Read the model definition and answer for the solid it produces. Units are mm, in the model's axes. Face numbers are marked on the shaded views. Round coordinates to 2 decimals unless told otherwise and drop trailing zeros. Order: outer loops, then holes, each group sorted by start corner. A loop starts at its lowest first (then second) coordinate and runs counter-clockwise, first axis right, second up.
from build123d import *

# Parameters (mm, degrees)
FILLET_1_R     = 2
FILLET_2_R     = 5
FILLET_3_R     = 7
CHAMFER_1_SIZE = 2
FILLET_4_R     = 1


with BuildPart() as part:
    # Эскиз1 → Повернуть1 (revolve)
    with BuildSketch(Plane.XY, mode=Mode.PRIVATE) as revolve_1_sk:
        Polygon((0, 20), (-11, 20), (-11, 50), (-15, 50), (-17.5, 19), (-22.5, 15), (-22.5, 0), (0, 0), align=None)
    revolve(revolve_1_sk.sketch.rotate(Axis((0, 0, 0), (0, 1, 0)), 270), axis=Axis((0, 0, 0), (0, 1, 0)))

    # Скругление1
    fillet_1_edges = [part.edges().sort_by_distance(p)[0] for p in [
        (0, 50, 15),
    ]]
    fillet(fillet_1_edges, radius=FILLET_1_R)

    # Скругление2
    fillet_2_edges = [part.edges().sort_by_distance(p)[0] for p in [
        (0, 19, 17.5),
    ]]
    fillet(fillet_2_edges, radius=FILLET_2_R)

    # Скругление3
    fillet_3_edges = [part.edges().sort_by_distance(p)[0] for p in [
        (0, 15, 22.5),
    ]]
    fillet(fillet_3_edges, radius=FILLET_3_R)

    # Фаска1
    chamfer_1_edges = [part.edges().sort_by_distance(p)[0] for p in [
        (0, 0, 22.5),
    ]]
    chamfer(chamfer_1_edges, length=CHAMFER_1_SIZE)

    # Скругление4
    fillet_4_edges = [part.edges().sort_by_distance(p)[0] for p in [
        (0, 20, 11),
    ]]
    fillet(fillet_4_edges, radius=FILLET_4_R)


solid = part.part
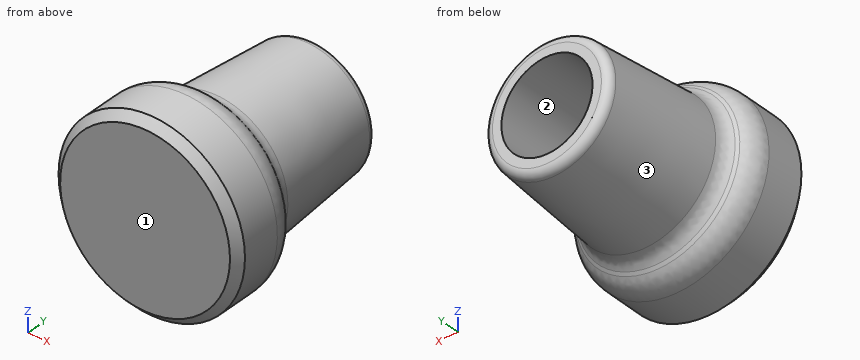
Q1. A cutting plane is placed at A-A, the plane y = 32. Give the vertices of the cut face in (x, z), plus the area to 3 significant figures.
Outcome:
outline: circle Ø32.9 at (0, 0); hole circle Ø22 at (0, 0)
area: 470 mm2
Q2. For a pull along X with two mould halves and no side action, classify the marked faces 1, 2 and 3 as released by +X, released by -X, zero draft, split by the parting line, or undercut.
Outcome:
face 1: zero draft
face 2: undercut
face 3: split by the parting line
Q3. Flat-ended cylindrical pins translate along their axes: pin 1 (5 mm diameter, centred on y = 21.5, z = 12.5, fed in from -X); pin 2 (4 mm diameter, centred on x = 13.5, y = 26.5, fed in from -Z); pin 3 (4 mm diameter, centred on y = 36.5, z = -11, fed in from -X). Find the tip coordinate at first contact, or state that the pin passes through.
Outcome:
pin 1: stops at x = -14.13
pin 2: stops at z = -12.39
pin 3: stops at x = -13.35
Q4. Straight lines are drawn through the part: probe 1 along Z at (x, y) = (-1.5, 40); probe 2 along Y at (x, z) = (2.5, -6.5); probe 3 along Z at (x, y) = (-9, 22). For each, find the intervals that lie inside material, in ascending order.
Outcome:
probe 1: z = -15.74 to -10.9, 10.9 to 15.74
probe 2: y = 0 to 20
probe 3: z = -14.73 to -6.32, 6.32 to 14.73
